from build123d import *

# Parameters (mm, degrees)
EXTRUDE_1_DEPTH          = 15
CUT_EXTRUDE_1_REACH      = 22
SKETCH_2_R               = 6
SKETCH_3_R               = 6
EXTRUDE_2_DEPTH          = 20
SKETCH_4_R               = 2.5
CUT_EXTRUDE_2_DEPTH      = 16
SKETCH_5_R               = 2.5
CUT_EXTRUDE_3_DEPTH      = 16.0000001
CUT_EXTRUDE_3_DEPTH_BACK = 16


with BuildPart() as part:
    # 草图1 → 凸台-拉伸1 (new body, symmetric)
    with BuildSketch(Plane.XY):
        Polygon((-40, 10), (0, 10), (0, 0), (30, 0), (30, -10), (-15, -10), (-15, 0), (-40, 0), align=None)
    extrude(amount=EXTRUDE_1_DEPTH, both=True)

    # 草图2 → 切除-拉伸1 (cut, up to next)
    with BuildSketch(Plane(origin=(0, 10, 0), x_dir=(1, 0, 0), z_dir=(0, 1, 0)), mode=Mode.PRIVATE) as cut_extrude_1_sk1:
        with Locations((-30, 0)):
            Circle(SKETCH_2_R)
    cut_extrude_1_tool1 = extrude(cut_extrude_1_sk1.sketch, amount=-CUT_EXTRUDE_1_REACH, mode=Mode.PRIVATE) & part.part
    add(cut_extrude_1_tool1.solids().sort_by_distance((-30, 10, 0))[0], mode=Mode.SUBTRACT)

    # 草图3 → 凸台-拉伸2 (add)
    with BuildSketch(Plane.XZ.offset(10)):
        with Locations((20, 0)):
            Circle(SKETCH_3_R)
    extrude(amount=EXTRUDE_2_DEPTH)

    # 草图4 → 切除-拉伸2 (cut, through all)
    with BuildSketch(Plane.XY):
        with Locations((-30, 5)):
            Circle(SKETCH_4_R)
    extrude(amount=-CUT_EXTRUDE_2_DEPTH, mode=Mode.SUBTRACT)

    # 草图5 → 切除-拉伸3 (cut, two sides)
    with BuildSketch(Plane(origin=(0, 0, 0), x_dir=(-1, 0, 0), z_dir=(0, 0, -1))) as cut_extrude_3_sk:
        with Locations((-20, -25)):
            Circle(SKETCH_5_R)
    extrude(amount=CUT_EXTRUDE_3_DEPTH, mode=Mode.SUBTRACT)
    extrude(cut_extrude_3_sk.sketch, amount=-CUT_EXTRUDE_3_DEPTH_BACK, mode=Mode.SUBTRACT)


solid = part.part
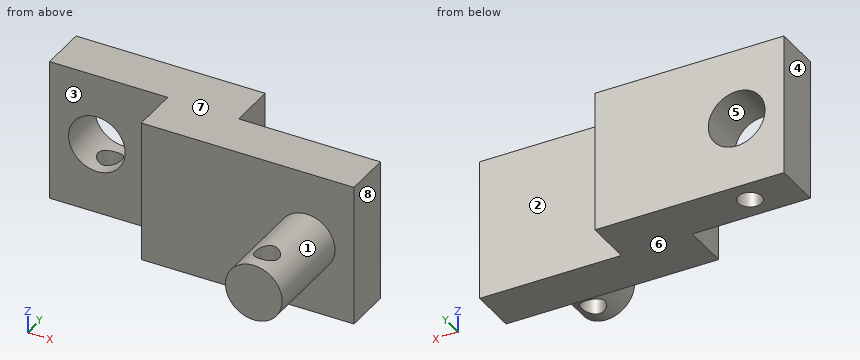
Input: part model. Units: mm. Frame: model coordinates. Face numbers are marked on the shaded views. A direction names the side the tool comes from. Give positions to 0.01 mm unless a question says otherwise; leave off trailing zeros. Loops run counter-clockwise (first coordinate to the right, second up) from the corner with the lowest first, then second, coordinate; pieces in that order, holes last. Notation, with made-up numbers: M 29.25,47.5 L 47.25,47.5 A13 ccw 47.25,62.5 Z; hole C 37.25,-17 d11. An arc over 180 degrees is marked long. Use one line per item in the form item = value.
1. Line query: L1, parallel to X at y = 5, z = -9.5; L2, parallel to Y at x = -30, z = -9.5; L3, parallel to X at y = 5.25, z = 0. Output: solid intervals per line, ascending.
Numbers:
L1 = -40 to -32.5, -27.5 to 0
L2 = 0 to 2.5, 7.5 to 10
L3 = -40 to -36, -24 to 0
2. Section query C-C, the plane z = -9.5. Return the cut outline in (x, y).
Numbers:
outline = M -40,0 L -15,0 L -15,-10 L 30,-10 L 30,0 L 0,0 L 0,10 L -40,10 Z; hole C -30,5 d5
3. Section query D-D, the plane y = 5. Return the cut outline in (x, z).
Numbers:
outline = M -40,-15 L -32.5,-15 L -32.5,-5.45 A6 cw long -27.5,-5.45 L -27.5,-15 L 0,-15 L 0,15 L -40,15 Z
4. Reachability of the marked faces 1, 2, 3 and 4 from +Z, -Z, +X, -X, +Y, -Y: full face, straight path, thin tool, end or side. Return the list, or none.
Numbers:
face_1 = -Y
face_2 = +Z, -Z, +X, +Y
face_3 = +Z, -Z, -X, -Y
face_4 = +Z, -Z, -X, +Y, -Y
5. Section query A-A, the plane z = 0. Return the cut outline in (x, y).
Numbers:
outline = M -40,0 L -36,0 L -36,10 L -40,10 Z; M -24,0 L -15,0 L -15,-10 L 14,-10 L 14,-30 L 26,-30 L 26,-10 L 30,-10 L 30,0 L 0,0 L 0,10 L -24,10 Z; hole C 20,-25 d5
6. First-contact query: pin 1 (4 mm diameter, centred on y = -4.5, z = -7.5, fed in from -X); pin 2 (4 mm diameter, centred on x = 16, y = -21.5, fed in from -Z); pin 3 (12.5 mm diameter, centred on x = -28, z = -2, fed in from -Y). Flat tips, straight axial feed; report the tip coordinate or a pass-through.
Numbers:
pin_1 = -15
pin_2 = -5.66
pin_3 = 0
7. Section query B-B, the plane x = 20. Return the cut outline in (y, z), and give its area (3 significant figures).
Numbers:
outline = M -30,-6 L -27.5,-6 L -27.5,6 L -30,6 Z; M -22.5,-6 L -10,-6 L -10,-15 L 0,-15 L 0,15 L -10,15 L -10,6 L -22.5,6 Z
area = 480 mm²
8. Pull-direction query (Z, two-part tool) for the marked faces 5, 6, 7 and 8; classes: released by +Z, released by -Z, zero draft, split by the parting line, or undercut.
Numbers:
face_5 = undercut
face_6 = released by -Z
face_7 = released by +Z
face_8 = zero draft
